The listing builds one solid part. Answer for the finished solid, in the listing's coordinates (mm). A direction names the side the tool comes from. Coordinates: 2 decimals unless noted, no trailing zeros. Write each loop counter-clockwise with the first axis right and the second up, starting at its lowest first coordinate (ties: lowest second). Pieces come first, ordered by that corner, then holes.
from build123d import *

# Parameters (mm, degrees)
PAD_DEPTH    = 10
SKETCH001_R  = 1.6
POCKET_DEPTH = 5
FILLET_R     = 1
FILLET001_R  = 4
FILLET002_R  = 1


with BuildPart() as part:
    # Sketch → Pad (new body)
    with BuildSketch(Plane.XZ):
        Polygon((0, 0), (0, 5), (8, 5), (8, 24), (25, 24), (25, 22), (10, 22), (10, 0), align=None)
    extrude(amount=PAD_DEPTH)

    # Sketch001 (on Face2 of Pad) → Pocket (cut)
    with BuildSketch(Plane(origin=(0, 0, 5), x_dir=(-1, 0, 0), z_dir=(0, 0, 1))):
        with Locations((-5, 5)):
            Circle(SKETCH001_R)
    extrude(amount=-POCKET_DEPTH, mode=Mode.SUBTRACT)

    # Fillet
    fillet_edges = [part.edges().sort_by_distance(p)[0] for p in [
        (8, -5, 5),
    ]]
    fillet(fillet_edges, radius=FILLET_R)

    # Fillet001
    fillet001_edges = [part.edges().sort_by_distance(p)[0] for p in [
        (0, 0, 2.5),
        (0, -10, 2.5),
    ]]
    fillet(fillet001_edges, radius=FILLET001_R)

    # Fillet002
    fillet002_edges = [part.edges().sort_by_distance(p)[0] for p in [
        (25, -5, 22),
    ]]
    fillet(fillet002_edges, radius=FILLET002_R)


solid = part.part
1. A tool of negligible diameter and unlimited length cuts with its end or side. For faces 1 (the flat face through (0, -5, 2)), 2 (the flat face through (17, -5, 22)), 3 (the flat face through (3, -5, 5)), from which of +Z, -Z, +X, -X, +Y, -Y can it reach the whole face along a straight path? Write none if from no direction.
Results found:
face 1: +Z, -Z, -X, +Y, -Y
face 2: -Z, +X, +Y, -Y
face 3: +Z, -X, +Y, -Y
2. Section D-D on y = -1.75 is taken. Give the vertices of the cut face in (x, z).
Results found:
outline: (0.69, 0) - (10, 0) - (10, 22) - (24, 22) arc R1 ccw to (25, 23) - (25, 24) - (8, 24) - (8, 6) arc R1 cw to (7, 5) - (0.69, 5) - close
3. Find the intervals of material crossed by L1, parallel to X at y = -5, z = 2.2; L2, parallel to Y at x = 5, z = 1.9; L3, parallel to Z at x = 21, y = -2.5, in increasing order.
Results found:
L1: x = 0 to 3.4, 6.6 to 10
L2: y = -10 to -6.6, -3.4 to 0
L3: z = 22 to 24
4. For a pull along X with two mould halves and no side action, classify faces 4 (the flat face through (8, -5, 15)), 5 (the flat face through (9, 0, 13)), 6 (the cylindrical face through (6.27, -4.03, 2.54)) as pulls with the +X half, pulls with the -X half, needs draft (parallel to the pull), parting line crosses it, or undercut.
Results found:
face 4: pulls with the -X half
face 5: needs draft
face 6: undercut
5. Section B-B on x = 5 is taken. Give the vertices of the cut face in (y, z).
Results found:
outline: (-10, 0) - (-6.6, 0) - (-6.6, 5) - (-10, 5) - close; (-3.4, 0) - (0, 0) - (0, 5) - (-3.4, 5) - close
6. Flat-ended cylindrical pins translate along their axes: P1, Ø5.5, axis at x = 3, y = -7, coming from the +Z side; P2, Ø3, axis at y = -7, z = 5.5, coming from the +X side; P3, Ø5, axis at y = -3, z = 13, coming from the -X side. Find the tip coordinate at first contact, or state that the pin passes through.
Results found:
P1: stops at z = 5
P2: stops at x = 10
P3: stops at x = 8
7. Section C-C on z = 16.5 is taken. Give the vertices of the cut face in (x, y).
Results found:
outline: (8, -10) - (10, -10) - (10, 0) - (8, 0) - close
8. Section A-A on y = -5 is taken. Give the vertices of the cut face in (x, z).
Results found:
outline: (0, 0) - (3.4, 0) - (3.4, 5) - (0, 5) - close; (6.6, 0) - (10, 0) - (10, 22) - (24, 22) arc R1 ccw to (25, 23) - (25, 24) - (8, 24) - (8, 6) arc R1 cw to (7, 5) - (6.6, 5) - close
